```python
from build123d import *

# Parameters (mm, degrees)
F0_R     = 12.7
F1_DEPTH = 3.1496
F2_R     = 6.9088
F3_DEPTH = 34.544
F4_R     = 5.6134
F5_DEPTH = 37.6946


with BuildPart() as f1:
    # F0 (on Front) → F1 (new body)
    with BuildSketch(Plane.XZ):
        Circle(F0_R)
    extrude(amount=F1_DEPTH)

    # F2 (on face) → F3 (join)
    with BuildSketch(Plane.XZ.offset(3.1496)):
        Circle(F2_R)
    extrude(amount=F3_DEPTH)

    # F4 (on face) → F5 (cut, through all)
    with BuildSketch(Plane(origin=(0, 0, 0), x_dir=(-1, 0, 0), z_dir=(0, 1, 0))):
        Circle(F4_R)
    extrude(amount=-F5_DEPTH, mode=Mode.SUBTRACT)


solid = f1.part
```
Could you check a few things on this model? Use its own coordinates, in mm. A direction names the side the tool comes from. Round coordinates to 2 decimals unless told otherwise and drop trailing zeros. Loops run counter-clockwise (first coordinate to the right, second up) from the corner with the lowest first, then second, coordinate; pieces in that order, holes last. Notation, with made-up numbers: (88, 34.25) - (101, 34.25) arc R8 ccw to (101, 49.25) - close; hole circle Ø4 at (8, 85). An arc over 180 degrees is marked (long way). Use CSV: the item, a comma, the result in double quotes.
Item 1: If we section it at D-D on z = 6.25: List the corners of the cut face in (x, y) for me.
Here are the results:
outline,"(-11.06, -3.15) - (-2.94, -3.15) - (-2.94, -37.69) - (2.94, -37.69) - (2.94, -3.15) - (11.06, -3.15) - (11.06, 0) - (-11.06, 0) - close"
Item 2: If we section it at C-C on y = -5: List the corners of the cut face in (x, z) for me, then the cut area to 3 significant figures.
Here are the results:
outline,"circle Ø13.82 at (0, 0); hole circle Ø11.23 at (0, 0)"
area,"51.0 mm²"
Item 3: Will these pins go through, and if not, where does the flat tip stop? pin 1 (3 mm diameter, centred on y = -31.5, z = 8.5, fed in from +X); pin 2 (10 mm diameter, centred on x = 3.5, y = -26.5, fed in from -Z); pin 3 (2 mm diameter, centred on y = -19.5, z = -3.5, fed in from +X); pin 4 (12 mm diameter, centred on y = -32.5, z = 6, fed in from -X).
Here are the results:
pin 1,"passes through"
pin 2,"stops at z = -6.91"
pin 3,"stops at x = 6.44"
pin 4,"stops at x = -6.91"
Item 4: I need wall thicknesses on L1, parallel to X at y = -11, z = 0.25; L2, parallel to Z at x = 0, y = -23; L3, parallel to Z at x = 4.5, y = -10. Which ranges of each line are inside material? Lowest first, please. Write a range as [from, to].
Here are the results:
L1,"x = [-6.9, -5.61], [5.61, 6.9]"
L2,"z = [-6.91, -5.61], [5.61, 6.91]"
L3,"z = [-5.24, -3.36], [3.36, 5.24]"
Item 5: If we section it at B-B on x = 0: List the corners of the cut face in (y, z) for me, then the cut area to 3 significant figures.
Here are the results:
outline,"(-37.69, -6.91) - (-3.15, -6.91) - (-3.15, -12.7) - (0, -12.7) - (0, -5.61) - (-37.69, -5.61) - close; (-37.69, 5.61) - (0, 5.61) - (0, 12.7) - (-3.15, 12.7) - (-3.15, 6.91) - (-37.69, 6.91) - close"
area,"134 mm²"
Item 6: If we section it at A-A on z = 0: List the corners of the cut face in (x, y) for me.
Here are the results:
outline,"(-12.7, -3.15) - (-6.91, -3.15) - (-6.91, -37.69) - (-5.61, -37.69) - (-5.61, 0) - (-12.7, 0) - close; (5.61, -37.69) - (6.91, -37.69) - (6.91, -3.15) - (12.7, -3.15) - (12.7, 0) - (5.61, 0) - close"
Item 7: If we mould it in two halves opening along Z, with no side actions, what happens to faces 1 (the cylindrical face through (1.22, -18.58, -5.48)), 2 (the flat face through (5, 0, -3)), 3 (the cylindrical face through (-2.75, -1.55, -12.4))? For each: pulls with the +Z half, pulls with the -Z half, needs draft (parallel to the pull), parting line crosses it, or undercut.
Here are the results:
face 1,"undercut"
face 2,"needs draft"
face 3,"parting line crosses it"
Item 8: For faces 4 (the cylindrical face through (-0.9, -20.18, 6.85)), 5 (the flat face through (0, -37.694, 6)), which set-ups out of +Z, -Z, +X, -X, +Y, -Y let a thin tool reach every point of the face, with its end or its side?
Here are the results:
face 4,"-Y"
face 5,"+Z, -Z, +X, -X, -Y"
